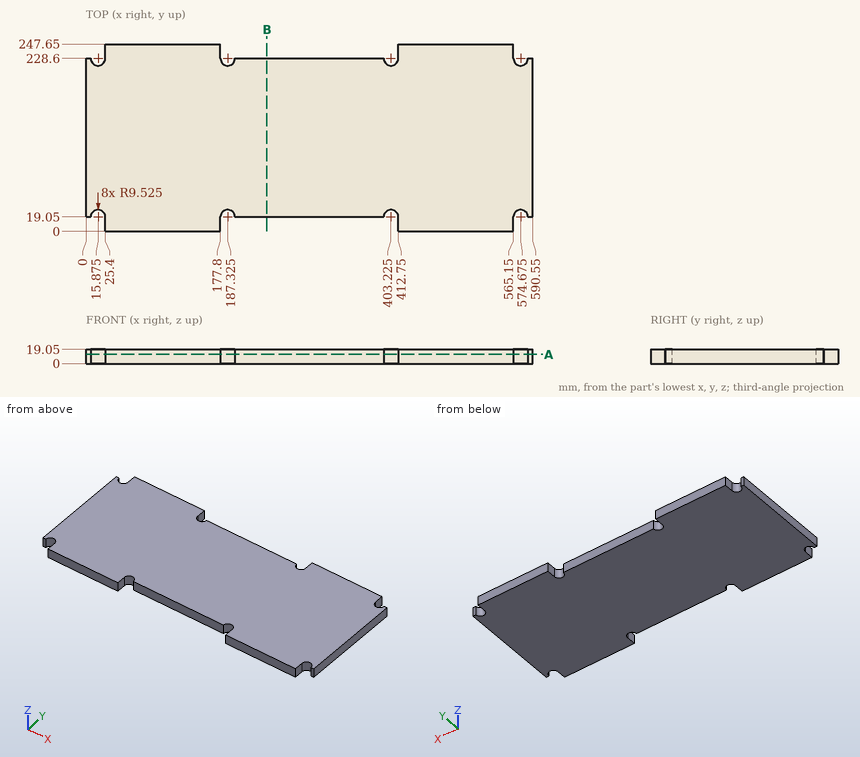
The drawing under review shows one solid part. Ordinate dimensions are in mm from its lowest x, y, z. Round coordinates to 2 decimals unless told otherwise and drop trailing zeros. Write each loop counter-clockwise with the first axis right and the second up, starting at its lowest first coordinate (ties: lowest second). Pieces come first, ordered by that corner, then holes. Notation, with made-up numbers: M -13,85.25 L 28,85.25 A20 ccw 28,89.25 Z; hole C 5.5,67 d6. An arc over 180 degrees is marked long. One line per item, written item: value. Start each with the question number.
(1) We need section B-B (x = 239). Give the boundary of the cut face in (y, z).
(2) Insertion check: pin 1 (7 mm diameter, centred on x = 589, z = 12, fed in from +Y); pin 2 (9.5 mm diameter, centred on y = 241, z = 5.5, fed in from -X); pin 3 (5.5 mm diameter, centred on x = 262.5, z = 9.5, fed in from -Y). Each pin has a flat end and moves straight along its axis. Give the tip position at first contact, or say it passes through.
(3) We need section A-A (z = 12.5). Give the boundary of the cut face in (x, y) (3 decimals).
(4) Wall thickness on line 1 (X direction, y = 232.5, z = 12.25); line 2 (Y direction, x = 313.5, z = 17.75); line 3 (Y direction, x = 195.5, z = 5): over which ranges is each line inside the solid? List them lowest first.
Result:
1. outline: M 19.05,0 L 228.6,0 L 228.6,19.05 L 19.05,19.05 Z
2. pin 1: y = 228.6
2. pin 2: x = 25.4
2. pin 3: y = 19.05
3. outline: M 0,19.05 L 6.35,19.05 A9.525 cw 25.4,19.05 L 25.4,0 L 177.8,0 L 177.8,19.05 A9.525 cw 196.85,19.05 L 393.7,19.05 A9.525 cw 412.75,19.05 L 412.75,0 L 565.15,0 L 565.15,19.05 A9.525 cw 584.2,19.05 L 590.55,19.05 L 590.55,228.6 L 584.2,228.6 A9.525 cw 565.15,228.6 L 565.15,247.65 L 412.75,247.65 L 412.75,228.6 A9.525 cw 393.7,228.6 L 196.85,228.6 A9.525 cw 177.8,228.6 L 177.8,247.65 L 25.4,247.65 L 25.4,228.6 A9.525 cw 6.35,228.6 L 0,228.6 Z
4. line 1: 25.4 to 177.8, 412.75 to 565.15
4. line 2: 19.05 to 228.6
4. line 3: 23.94 to 223.71
